Autodesk Inventor part; units mm, degrees
ref_plane "YZ Plane" through (0, 0, 0) normal (1, 0, 0) x (0, 1, 0)
ref_plane "XZ Plane" through (0, 0, 0) normal (0, 1, 0) x (-1, 0, 0)
ref_plane "XY Plane" through (0, 0, 0) normal (0, 0, 1) x (1, 0, 0)
sketch "Sketch1" plane through (0, 0, 0) normal (0, 1, 0) x (-1, 0, 0)
  line L0 (-10, -11.1404) -> (10, -11.1404)
  line L1 (10, -11.1404) -> (10, 18.8596)
  line L2 (10, 18.8596) -> (-10, 18.8596)
  line L3 (-10, 18.8596) -> (-10, -11.1404)
  point P0 (0, 0)
  dimension "d0" = 20
  dimension "d1" = 10
  dimension "d2" = 30
extrude "Extrusion1" add sketch "Sketch1" along normal blind 0.2
sketch "Sketch2" plane through (10, 0, 18.8596) normal (1, 0, 0) x (0, 0, -1)
  line L0 (30, 0.2) -> (0, 0.2)
  arc A0 (0, 0.2) -> (-1, -0.8) centre (0, -0.8) ccw
  line L1 (0, -0.8) -> (-1, -0.8) construction
  line L2 (0, -0.8) -> (0, 0.2) construction
  arc A1 (0, 0) -> (-0.8, -0.8) centre (0, -0.8) ccw
  line L3 (0, 0) -> (30, 0)
  line L4 (-0.8, -0.8) -> (-0.8, -15.8)
  line L5 (-0.8, -15.8) -> (-1, -15.8)
  line L6 (-1, -15.8) -> (-1, -0.8)
  line L7 (0, 0) -> (0, 0.2)
  point P0 (18.8596, 0)
  dimension "d5" = 90
  dimension "d6" = 1
  dimension "d7" = 0.2
  dimension "d8" = 0.2
  dimension "d9" = 15
extrude "Extrusion2" add sketch "Sketch2" against normal up to surface (20 mm away)
sketch "Sketch3" plane through (10, -15.8, 19.8596) normal (1, 0, 0) x (0, 0, -1)
  arc A0 (1, 16) -> (0, 15) centre (1, 15) ccw
  arc A1 (1, 15.8) -> (0.2, 15) centre (1, 15) ccw
  line L0 (0, 13.8) -> (0.2, 13.8)
  line L1 (0, 15) -> (0, 0)
  line L2 (0.2, 0) -> (0.2, 15)
  line L3 (0, 0) -> (0.2, 0)
  point P0 (19.8596, 15.8)
  dimension "d19" = 1.2
extrude "Extrusion3" add sketch "Sketch3" along normal blind 52.7
sketch "Sketch4" plane through (10, -2, 19.8596) normal (0, 1, 0) x (1, 0, 0)
  line L0 (52.7, 0.2) -> (52.7, 0)
  arc A0 (52.7, 0) -> (53.7, 1) centre (52.7, 1) ccw
  line L1 (52.7, 1) -> (53.7, 1) construction
  line L2 (52.7, 1) -> (52.7, 0) construction
  arc A1 (52.7, 0.2) -> (53.5, 1) centre (52.7, 1) ccw
  line L3 (53.5, 1) -> (53.5, 47)
  line L4 (53.5, 47) -> (53.7, 47)
  line L5 (53.7, 47) -> (53.7, 1)
  point P0 (-10, 19.8596)
  dimension "d14" = 90
  dimension "d15" = 1
  dimension "d16" = 46
  dimension "d28" = 0.2
extrude "Extrusion4" add sketch "Sketch4" against normal up to surface (13.8 mm away)
sketch "Sketch5" plane through (63.7, -2, 18.8596) normal (1, 0, 0) x (0, 0, -1)
  line L0 (46, 0) -> (0, 0)
  line L1 (0, 0) -> (0, 0)
  line L2 (46, 0) -> (46, 7.5)
  line L3 (46, 7.5) -> (5, 7.5)
  line L4 (5, 7.5) -> (5, 5)
  arc A0 (0, 0) -> (5, 5) centre (0, 5) ccw
  point P0 (18.8596, 2)
  point P1 (5, 6.25)
  point P2 (30, 0)
  dimension "d20" = 7.5
  dimension "d21" = 5
  dimension "d22" = 5
extrude "Extrusion5" add sketch "Sketch5" against normal up to surface (0.2 mm away)
sketch "Sketch6" plane through (63.7, -15.8, 18.8596) normal (1, 0, 0) x (0, 0, -1)
  line L0 (46, 0) -> (46, 21.3)
  line L1 (46, 0) -> (5, 0)
  line L2 (5, -3.2119) -> (46, -3.2119)
  line L3 (46, -3.2119) -> (46, 0)
  line L4 (5, 21.3) -> (5, 18.8)
  line L5 (46, 0) -> (0, 0)
  arc A0 (5, -3.2119) -> (0, 0) centre (0, -5.4977) ccw
  line L6 (-1, 0) -> (0, 0)
  line L7 (0, 0) -> (5, 0)
  point P0 (18.8596, 15.8)
  point P1 (46.1737, 13.8)
extrude "Extrusion6" add sketch "Sketch6" against normal up to surface (0.2 mm away)
fillet "Fillet1" radius 1 8 edges at (63.6, 5.5, 13.8596) (63.6, 5.5, -27.1404) (63.6, -19.0119, -27.1404) (63.6, -19.0119, 13.8596) (10, 0.1, -11.1404) (-10, 0.1, -11.1404) (-10, -15.8, 19.7596) (10, -2, 19.7596)
sketch "Sketch7" plane through (0, 0.2, 0) normal (0, 1, 0) x (1, 0, 0)
  line L0 (-10, 10.1404) -> (-10, -18.8596)
  line L1 (9, 11.1404) -> (-9, 11.1404)
  line L2 (10, -18.8596) -> (10, 10.1404)
  point P0 (0, 0)
  point P1 (7.5, 8.6404)
  point P2 (-7.5, 8.6404)
  dimension "d29" = 2.5
  dimension "d30" = 2.5
  dimension "d31" = 2.5
hole "Hole1" at (7.5, 0.2, -8.6404) at (-7.5, 0.2, -8.6404) direction (0, -1, 0) diameter 2 depth 7.9 tip angle 118
sketch "Sketch8" plane through (63.7, -15.8, 18.8596) normal (1, 0, 0) x (0, 0, -1)
  line L0 (45, 21.3) -> (6, 21.3)
  line L1 (5.6057, -3.2119) -> (45, -3.2119)
  line L2 (46, -2.2119) -> (46, 20.3)
  point P0 (18.8596, 15.8)
  point P1 (18.26, 9.044)
  point P2 (33.26, 9.044)
  dimension "d39" = 24.5119
  dimension "d40" = 12.256
  dimension "d41" = 15
  dimension "d42" = 12.74
hole "Hole2" at (63.7, -6.756, 0.5996) at (63.7, -6.756, -14.4004) direction (-1, 0, 0) diameter 3.4 depth 7.9 tip angle 118
equation "\"d8\" = d7"
properties part number "Flex V1" material "Copper"
Read the model definition and answer for the solid it produces. Units are mm, in the model's axes. A direction names the side the tool comes from. Round coordinates to 2 decimals unless told otherwise and drop trailing zeros. Loops run counter-clockwise (first coordinate to the right, second up) from the corner with the lowest first, then second, coordinate; pieces in that order, holes last. Notation, with made-up numbers: (3, -4.5) - (61, -4.5) arc R18 cw to (61, 0.5) - close; hole circle Ø1 at (26.25, 85). An arc over 180 degrees is marked (long way). One line per question, with ' | ' between items. Start each with the question number.
Q1. Flat-ended cylindrical pins translate along their axes: pin 1 (22 mm diameter, centred on x = 0.5, z = 10, fed in from -Y); pin 2 (7.5 mm diameter, centred on y = -12.5, z = 1, fed in from -X); pin 3 (10 mm diameter, centred on x = 21.5, z = 12, fed in from +Y); pin 4 (0.5 mm diameter, centred on x = 30.5, z = 19.5, fed in from +Y). Find the tip coordinate at first contact, or state that the pin passes through.
Q2. For faces 1 (the flat face through (63.7, -7, -4)), 2 (the flat face through (0, 0.2, 4)), 3 (the flat face through (0, 0, 4)), determine the directions among +Z, -Z, +X, -X, +Y, -Y from which every point of the face is accessible in a straight line to the end or side of a thin tool.
Q3. Section B-B on z = 16 is taken. Give the vertices of the cut face in (x, y), plus the area to 3 significant figures.
Q4. Section A-A on x = -7.5 is taken. Give the vertices of the cut face in (y, z).
Q5. Section C-C on x = 4 is taken. Give the vertices of the cut face in (y, z), plus the area to 3 significant figures.
Q6. Section D-D on y = -11.25 is taken. Give the vertices of the cut face in (x, z).
Q7. Find the intervals of material crossed by L1, parallel to X at y = -16.25, z = 13.5; L2, parallel to Z at x = 28, y = -12; L3, parallel to Z at x = 7.5, y = 0.1, in increasing order.
Established:
1) pin 1: y = -15.8 | pin 2: x = 63.5 | pin 3: through | pin 4: y = -2
2) face 1: +Z, -Z, +X, +Y, -Y | face 2: +Z, -Z, -X, +Y | face 3: -Z, -X, -Y
3) outline: (-10, 0) - (10, 0) - (10, 0.2) - (-10, 0.2) - close; (63.5, -16.6) - (63.7, -16.6) - (63.7, -1.1) - (63.5, -1.1) - close | area: 7.10 mm²
4) outline: (-15.8, 19.66) - (-0.8, 19.66) arc R0.8 cw to (0, 18.86) - (0, -7.64) - (0.2, -7.64) - (0.2, 18.86) arc R1 ccw to (-0.8, 19.86) - (-15.8, 19.86) - close; (0, -11.14) - (0.2, -11.14) - (0.2, -9.64) - (0, -9.64) - close
5) outline: (-15.8, 19.66) - (-0.8, 19.66) arc R0.8 cw to (0, 18.86) - (0, -11.14) - (0.2, -11.14) - (0.2, 18.86) arc R1 ccw to (-0.8, 19.86) - (-15.8, 19.86) - close | area: 9.28 mm²
6) outline: (-10, 19.66) - (62.7, 19.66) arc R0.8 cw to (63.5, 18.86) - (63.5, -27.14) - (63.7, -27.14) - (63.7, 18.86) arc R1 ccw to (62.7, 19.86) - (-10, 19.86) - close
7) L1: 63.5 to 63.7 | L2: 19.66 to 19.86 | L3: -11.14 to -9.64, -7.64 to 19.3
